Here's the drawing with two shaded views (mm, measured from the low corner). I have some questions. Round coordinates to 2 decimals unless told otherwise and drop trailing zeros. Order: outer loops, then holes, each group sorted by start corner. A loop starts at its lowest first (then second) coordinate and runs counter-clockwise, first axis right, second up. Notation, with made-up numbers: (77.25, 18) -> (118.25, 18) arc R22 cw to (118.25, 27) -> close; hole circle Ø9 at (40, -26.75). An arc over 180 degrees is marked (long way). Answer in a Markdown table with one row per item.
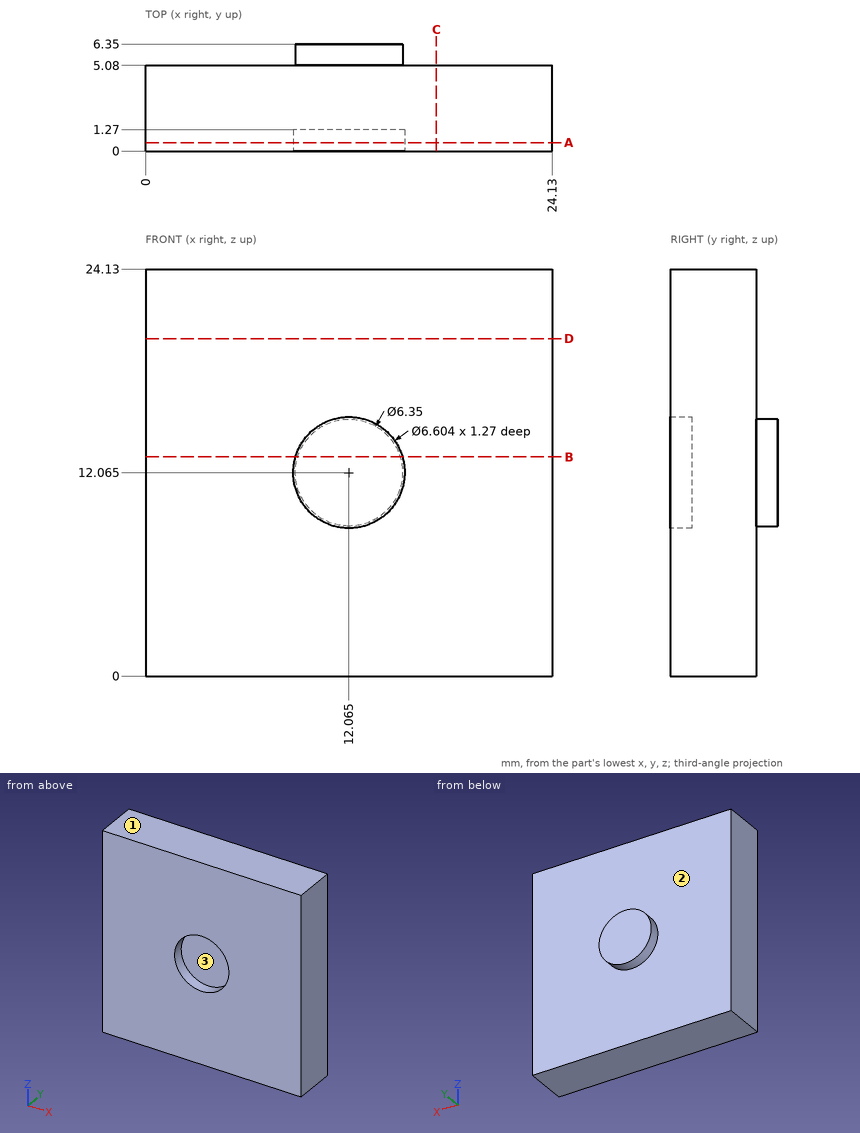
1. Please list where these lines run through material, in increasing order: line 1 along Y through (x, z) = (14.5, 12.75); line 2 along Y through (x, z) = (13.5, 3.75).
Numbers:
| item | result |
|---|---|
| line 1 | y = 1.27 to 6.35 |
| line 2 | y = 0 to 5.08 |
2. We'd pull the mould along Z, two halves only. Please class the marked faces 1, 2 and 3: released by +Z, released by -Z, zero draft, split by the parting line, or undercut.
Numbers:
| item | result |
|---|---|
| face 1 | released by +Z |
| face 2 | zero draft |
| face 3 | undercut |
3. For pin 1 Ø8 at (x, z) = (9.5, 3) entering from +Y; pin 2 Ø2 at (x, z) = (11.5, 12.5) entering from -Y, each with a flat end and sliding along its axis, tell me the tip position at first contact or that it passes through.
Numbers:
| item | result |
|---|---|
| pin 1 | stops at y = 5.08 |
| pin 2 | stops at y = 1.27 |
4. Suppose I cut it at D-D on z = 20. Write out the boundary of the cut face in (x, y).
Numbers:
| item | result |
|---|---|
| outline | (0, 0) -> (24.13, 0) -> (24.13, 5.08) -> (0, 5.08) -> close |
5. Suppose I cut it at B-B on z = 13. Write out the boundary of the cut face in (x, y), then the cut area to 3 significant figures.
Numbers:
| item | result |
|---|---|
| outline | (0, 0) -> (8.9, 0) -> (8.9, 1.27) -> (15.23, 1.27) -> (15.23, 0) -> (24.13, 0) -> (24.13, 5.08) -> (15.1, 5.08) -> (15.1, 6.35) -> (9.03, 6.35) -> (9.03, 5.08) -> (0, 5.08) -> close |
| area | 122 mm2 |
6. Suppose I cut it at C-C on x = 17.25. Write out the boundary of the cut face in (y, z), then the cut area to 3 significant figures.
Numbers:
| item | result |
|---|---|
| outline | (0, 0) -> (5.08, 0) -> (5.08, 24.13) -> (0, 24.13) -> close |
| area | 123 mm2 |
7. Suppose I cut it at A-A on y = 0.5. Write out the boundary of the cut face in (x, z) (3 decimals), then the cut area to 3 significant figures.
Numbers:
| item | result |
|---|---|
| outline | (0, 0) -> (24.13, 0) -> (24.13, 24.13) -> (0, 24.13) -> close; hole circle Ø6.604 at (12.065, 12.065) |
| area | 548 mm2 |
